Autodesk Inventor part; units mm, degrees
ref_plane "YZ Plane" through (0, 0, 0) normal (1, 0, 0) x (0, 1, 0)
ref_plane "XZ Plane" through (0, 0, 0) normal (0, 1, 0) x (-1, 0, 0)
ref_plane "XY Plane" through (0, 0, 0) normal (0, 0, 1) x (1, 0, 0)
sketch "Sketch1" plane through (0, 0, 0) normal (0, 1, 0) x (-1, 0, 0)
  line L0 (0, 0) -> (60, 0)
  line L1 (60, 0) -> (60, -120)
  line L2 (60, -120) -> (0, -120)
  line L3 (0, -120) -> (0, 0)
  dimension "d0" = 60
  dimension "d1" = 120
extrude "Extrusion1" add sketch "Sketch1" along normal blind 5
sketch "Sketch3" plane through (-60, 0, 0) normal (0, 0, 1) x (1, 0, 0)
  line L0 (0, 0) -> (60, 0)
  circle A0 centre (38.75, 11) radius 1.55
  circle A1 centre (21.25, 11) radius 1.55
  dimension "d22" = 3.1
  dimension "d23" = 3.1
  dimension "d25" = 17.5
  dimension "d26" = 11
  dimension "d27" = 11
extrude "Extrusion3" cut sketch "Sketch3" against normal through all
sketch "Sketch5" plane through (0, 5, 0) normal (0, 1, 0) x (1, 0, 0)
  line L0 (0, 0) -> (0, 120)
  line L1 (0, 120) -> (0, 108)
  line L2 (0, 108) -> (-7, 108)
  line L3 (-60, 120) -> (-60, 0)
  circle A0 centre (-7, 108) radius 1.55
  line L4 (0, 120) -> (-60, 120)
  line L5 (-30, 120) -> (-30, 0)
  line L6 (-45, 0) -> (-15, 0)
  line L7 (0, 60) -> (-60, 60)
  circle A1 centre (-53, 108) radius 1.55
  circle A2 centre (-7, 12) radius 1.55
  circle A3 centre (-53, 12) radius 1.55
  dimension "d47" = 12
  dimension "d48" = 7
  dimension "d49" = 3.1
extrude "Extrusion5" cut sketch "Sketch5" against normal blind 10 contours A0 | A1 | A2 | A3
sketch "Sketch7" plane through (0, 5, 0) normal (0, 1, 0) x (1, 0, 0)
  circle A0 centre (-18, 75) radius 2.45
  circle A1 centre (-42, 75) radius 2.45
  circle A2 centre (-42, 35) radius 2.45
  circle A3 centre (-18, 35) radius 2.45
  circle A4 centre (-18, 35) radius 1.55
  circle A5 centre (-42, 35) radius 1.55
  circle A6 centre (-18, 75) radius 1.55
  circle A7 centre (-42, 75) radius 1.55
  point P0 (0, 0)
  dimension "d64" = 3.1
  dimension "d65" = 3.1
  dimension "d66" = 3.1
  dimension "d67" = 3.1
extrude "Extrusion7" cut sketch "Sketch7" against normal blind 10 contours A4 | A5 | A6 | A7
properties part number "bottom_plate" material "PET Plastic"
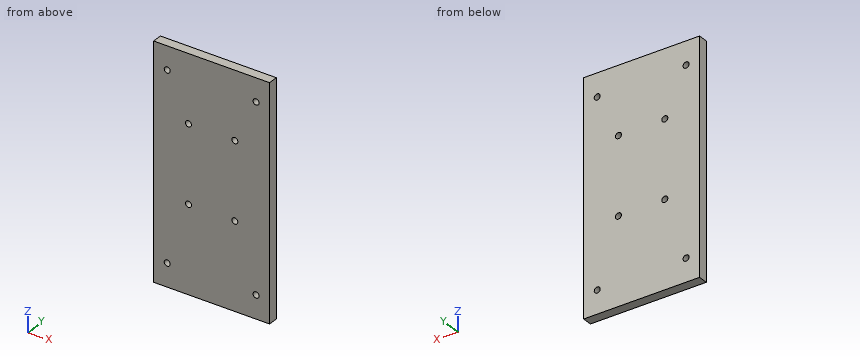
Here's how the part is built. I have some questions about the finished solid (model axes, mm). Coordinates: 2 decimals unless noted, no trailing zeros. Order: outer loops, then holes, each group sorted by start corner. A loop starts at its lowest first (then second) coordinate and runs counter-clockwise, first axis right, second up. Notation, with made-up numbers: M 46.25,57.25 L 60.25,57.25 A21 cw 60.25,92.25 Z; hole C 63,-6.75 d1. An arc over 180 degrees is marked long. Answer as a JSON object with one key per item and string values. Group by question number.
(1) Suppose I cut it at A-A, the plane z = -108. Please give me the cut outline in (x, y).
(2) For pin 1 (3 mm diameter, centred on x = -18, z = -75, fed in from +Y), with a flat end and sliding along its axis, tell me the tip position at first contact or that it passes through.
(3) I need wall thicknesses on probe 1 along X at (y, z) = (4, -35); probe 2 along Z at (x, y) = (-53, 2.15); probe 3 along Z at (x, y) = (-42, 3.65). Which ranges of each line are inside material? Lowest first, please.
(4) Suppose I cut it at B-B, the plane x = -7. Please give me the cut outline in (y, z).
Values found:
{
 "1": {"outline": "M -60,0 L -54.55,0 L -54.55,5 L -60,5 Z; M -51.45,0 L -8.55,0 L -8.55,5 L -51.45,5 Z; M -5.45,0 L 0,0 L 0,5 L -5.45,5 Z"},
 "2": {"pin 1": "passes through"},
 "3": {"probe 1": "x = -60 to -43.55, -40.45 to -19.55, -16.45 to 0", "probe 2": "z = -120 to -109.55, -106.45 to -13.55, -10.45 to 0", "probe 3": "z = -120 to -76.55, -73.45 to -36.55, -33.45 to 0"},
 "4": {"outline": "M 0,-120 L 5,-120 L 5,-109.55 L 0,-109.55 Z; M 0,-106.45 L 5,-106.45 L 5,-13.55 L 0,-13.55 Z; M 0,-10.45 L 5,-10.45 L 5,0 L 0,0 Z"}
}
